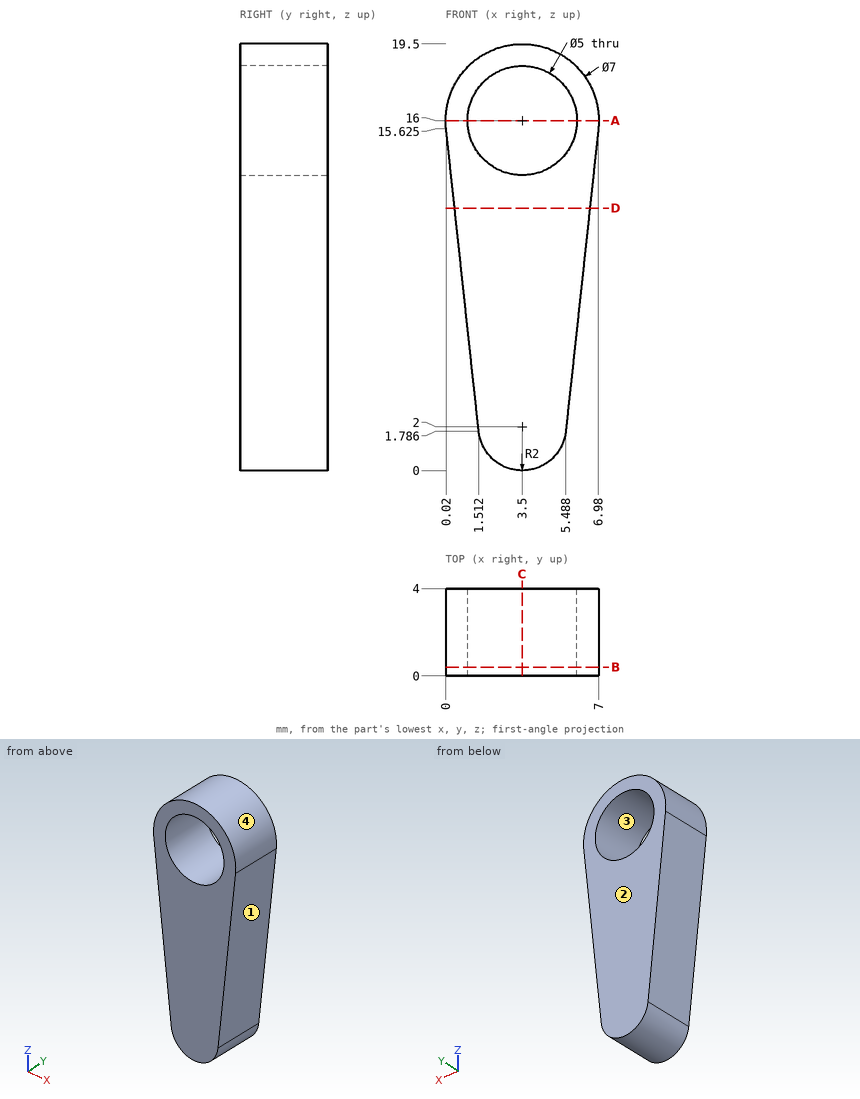
Geometry check sheet. Reference: drawing and pictorial views, mm from the part's lowest x, y, z. Coordinates: 2 decimals unless noted, no trailing zeros. Order: outer loops, then holes, each group sorted by start corner. A loop starts at its lowest first (then second) coordinate and runs counter-clockwise, first axis right, second up. Notation, with made-up numbers: M 61.25,-35.75 L 89.25,-35.75 A15 cw 89.25,-22.75 Z; hole C 56.25,-1 d2. An arc over 180 degrees is marked long. Return JSON: item names as keys, results as strings.
1) Release check for a two-part mould opening along X. For the marked faces 1, 2, 3 and 4 record: +X half, -X half, draft (parallel to the pull), parting line (faces both ways), or undercut.
Answer list:
{"face 1": "+X half", "face 2": "draft", "face 3": "undercut", "face 4": "parting line"}
2) Cross-section at A-A, the plane z = 16. Record the boundary of the cut face in (x, y).
Answer list:
{"outline": "M 0,0 L 1,0 L 1,4 L 0,4 Z; M 6,0 L 7,0 L 7,4 L 6,4 Z"}
3) Cross-section at C-C, the plane x = 3.5. Record the boundary of the cut face in (y, z), and give its area (3 significant figures).
Answer list:
{"outline": "M 0,0 L 4,0 L 4,13.5 L 0,13.5 Z; M 0,18.5 L 4,18.5 L 4,19.5 L 0,19.5 Z", "area": "58.0 mm2"}
4) Gauge pin test, flat ends, axial feed: pin 1 (4 mm diameter, centred on x = 3.5, z = 16, fed in from +Y); pin 2 (1 mm diameter, centred on y = 1.5, z = 14, fed in from +X). Record the tip position at first contact, or that the pin passes through.
Answer list:
{"pin 1": "through", "pin 2": "x = 6.86"}
5) Cross-section at D-D, the plane z = 12. Record the boundary of the cut face in (x, y), and give its area (3 significant figures).
Answer list:
{"outline": "M 0.41,0 L 6.59,0 L 6.59,4 L 0.41,4 Z", "area": "24.7 mm2"}
6) Cross-section at B-B, the plane y = 0.4. Record the boundary of the cut face in (x, z) (1 decimal).
Answer list:
{"outline": "M 0,15.6 L 1.5,1.8 A2 ccw 5.5,1.8 L 7,15.6 A3.5 ccw long Z; hole C 3.5,16 d5"}
7) Thickness scan on L1, parallel to X at y = 1.75, z = 16; L2, parallel to Z at x = 5, y = 2.2 (1 decimal); L3, parallel to Z at x = 4.5, y = 2.75 (1 decimal). Record the ranges inside material, lowest first. Write a range as [from, to].
Answer list:
{"L1": "[0, 1], [6, 7]", "L2": "[0.7, 14], [18, 19.2]", "L3": "[0.3, 13.7], [18.3, 19.4]"}
